The listing builds one solid part. Answer for the finished solid, in the listing's coordinates (mm). A direction names the side the tool comes from. Give positions to 0.01 mm unless a question says otherwise; leave off trailing zeros. Loops run counter-clockwise (first coordinate to the right, second up) from the corner with the lowest first, then second, coordinate; pieces in that order, holes last. Notation, with made-up numbers: M -4,55 L 50,55 A26 cw 50,69 Z; hole C -29.75,30 d9. An arc over 180 degrees is marked long. Use one line per item in the form item = value. Start each with the question number.
1. The part is cut by section C-C (z = 1.9). Write down the section's boundary in (x, y), and give its area (3 significant figures).
2. The part is cut by section A-A (y = 0.5). Write down the section's boundary in (x, z), and give its area (3 significant figures).
3. Straight lines are drawn through the part: line 1 (Y direction, x = -8, z = 0.7); line 2 (X direction, y = 0.25, z = 3.65). For each, find the intervals that lie inside material, in ascending order. Write a range as from..to.
4. For faces 1 (the face through (-10, 0, 1)), 2 (the face through (8.5, -0.1, 4.5)), 3 (the face through (0, 9.75, 2)), 4 (the face through (9.25, 0, 2)), 5 (the face through (0, -9.75, 2)), determine the directions among +Z, -Z, +X, -X, +Y, -Y from which every point of the face is accessible in a straight line to the end or side of a thin tool.
5. The mould has two halves that part along Y. Classify faces 6 (the face through (-9.465, 0.13, 4.699)), 7 (the face through (0.13, 9.465, 4.699)), 8 (the face through (-8.5, 0.1, 4.5)): released by +Y, released by -Y, zero draft, split by the parting line, or undercut.
6. Each of these flat-tipped pins is pushed along its axis until it touches: pin 1 Ø2 at (x, z) = (1.5, 2.5) entering from +Y; pin 2 Ø1.5 at (x, y) = (-8, 1) entering from -Z; pin 3 Ø1.1 at (y, z) = (-3, 4.5) entering from +X. Where does it stop, or does it pass through?
Autodesk Fusion 360 part; units mm, degrees
sketch "Sketch1" plane through (0, 0, 0) normal (0, 0, 1) x (1, 0, 0)
  line L0 (9.75, -9.75) -> (-9.75, -9.75)
  line L1 (-9.75, -9.75) -> (-9.75, 9.75)
  line L2 (-9.75, 9.75) -> (9.75, 9.75)
  line L3 (9.75, 9.75) -> (9.75, -9.75)
  line L4 (9.75, -9.75) -> (-9.75, 9.75) construction
  line L5 (-9.75, -9.75) -> (9.75, 9.75) construction
  line L6 (11.5, 11.5) -> (-11.5, 11.5)
  line L7 (-11.5, 11.5) -> (-11.5, -11.5)
  line L8 (-11.5, -11.5) -> (11.5, -11.5)
  line L9 (11.5, -11.5) -> (11.5, 11.5)
  line L10 (11.5, 11.5) -> (-11.5, -11.5) construction
  line L11 (-11.5, 11.5) -> (11.5, -11.5) construction
  line L12 (9.25, -9.25) -> (-9.25, -9.25)
  line L13 (-9.25, -9.25) -> (-9.25, 9.25)
  line L14 (-9.25, 9.25) -> (9.25, 9.25)
  line L15 (9.25, 9.25) -> (9.25, -9.25)
  line L16 (9.25, -9.25) -> (-9.25, 9.25) construction
  line L17 (-9.25, -9.25) -> (9.25, 9.25) construction
  dimension "d1" = 19.5
  dimension "d2" = 19.5
  dimension "d3" = 23
  dimension "d4" = 23
  dimension "d5" = 18.5
  dimension "d6" = 18.5
extrude "Extrude1" add sketch "Sketch1" along normal blind 1 contours L0 L1 L2 L3 | L6 L7 L8 L9 makes body 1
extrude "Extrude2" add sketch "Sketch1" along normal blind 5 contours L12 L13 L14 L15 bodies 1
sketch "Sketch2" plane through (0, 0, 5) normal (0, 0, 1) x (-1, 0, 0)
  line L0 (-9.25, -9.25) -> (9.25, -9.25)
  line L1 (9.25, -9.25) -> (9.25, 9.25)
  line L2 (9.25, 9.25) -> (-9.25, 9.25)
  line L3 (-9.25, 9.25) -> (-9.25, -9.25)
  line L4 (8.5, 8.5) -> (-8.5, 8.5)
  line L5 (-8.5, 8.5) -> (-8.5, -8.5)
  line L6 (-8.5, -8.5) -> (8.5, -8.5)
  line L7 (8.5, -8.5) -> (8.5, 8.5)
  line L8 (8.5, 8.5) -> (-8.5, -8.5) construction
  line L9 (-8.5, 8.5) -> (8.5, -8.5) construction
  dimension "d11" = 17
  dimension "d12" = 17
extrude "Extrude3" cut sketch "Sketch2" against normal blind 10 contours L4 L5 L6 L7 bodies 1
extrude "Extrude4" cut sketch "Sketch1" along normal blind 4 contours L12 L13 L14 L15 bodies 1 makes body 2 at (-2.8333, 9, 4)
extrude "Extrude5" add sketch "Sketch1" along normal blind 5 contours L0 L1 L2 L3 bodies 1 2
fillet "Fillet1" radius 0.5 12 edges at (-9.75, -9.75, 3) (-9.75, 9.75, 3) (9.75, 9.75, 3) (9.75, -9.75, 3) (11.5, 11.5, 0.5) (-11.5, 11.5, 0.5) (11.5, -11.5, 0.5) (-11.5, -11.5, 0.5) (0, -11.5, 0) (11.5, 0, 0) (0, 11.5, 0) (-11.5, 0, 0) on bodies 1
fillet "Fillet2" radius 1 8 edges at (9.6036, 9.6036, 5) (0, 9.75, 5) (-9.6036, 9.6036, 5) (-9.75, 0, 5) (-9.6036, -9.6036, 5) (0, -9.75, 5) (9.6036, -9.6036, 5) (9.75, 0, 5) on bodies 1
Derived:
q1.outline = M -9.75,-9.25 A0.5 ccw -9.25,-9.75 L 9.25,-9.75 A0.5 ccw 9.75,-9.25 L 9.75,9.25 A0.5 ccw 9.25,9.75 L -9.25,9.75 A0.5 ccw -9.75,9.25 Z; hole M -9.25,-9.25 L 9.25,-9.25 L 9.25,9.25 L -9.25,9.25 Z
q1.area = 37.8 mm2
q2.outline = M -11.5,0.5 A0.5 ccw -11,0 L -9.25,0 L -9.25,4 L -8.5,4 L -8.5,5 L -8.75,5 A1 ccw -9.75,4 L -9.75,1 L -11.5,1 Z; M 8.5,4 L 9.25,4 L 9.25,0 L 11,0 A0.5 ccw 11.5,0.5 L 11.5,1 L 9.75,1 L 9.75,4 A1 ccw 8.75,5 L 8.5,5 Z
q2.area = 9.46 mm2
q3.line_1 = -11.5..-9.25, 9.25..11.5
q3.line_2 = -9.75..-9.25, 9.25..9.75
q4.face_1 = +Z
q4.face_2 = +Z, -Z
q4.face_3 = +Z, +X, -X, +Y
q4.face_4 = -Z
q4.face_5 = +Z, +X, -X, -Y
q5.face_6 = zero draft
q5.face_7 = released by +Y
q5.face_8 = undercut
q6.pin_1 = 9.75
q6.pin_2 = 4
q6.pin_3 = 9.75
